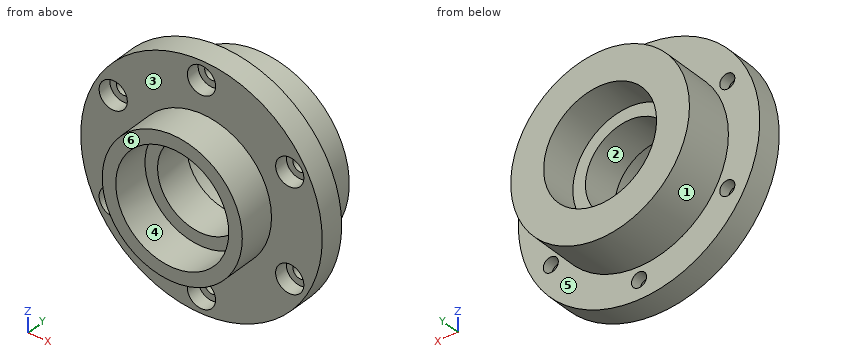
from build123d import *

# Parameters (mm, degrees)
F0_R            = 30.5435
F1_DEPTH        = 6.35
F2_R            = 17.7165
F2_R_2          = 14.2875
F3_DEPTH        = 9.525
F4_R            = 22.606
F5_DEPTH        = 12.7
F6_R            = 14.2875
F7_DEPTH        = 9.525
F8_R            = 11.1125
F9_DEPTH        = 19.05
F11_D           = 3.81
F11_CBORE_D     = 7.1374
F11_CBORE_DEPTH = 3.5052


with BuildPart() as f1:
    # F0 (on Front) → F1 (new body)
    with BuildSketch(Plane.XZ):
        Circle(F0_R)
    extrude(amount=F1_DEPTH)

    # F2 (on face) → F3 (join)
    with BuildSketch(Plane.XZ.offset(6.35)):
        Circle(F2_R)
        Circle(F2_R_2, mode=Mode.SUBTRACT)
    extrude(amount=F3_DEPTH)

    # F4 (on face) → F5 (join)
    with BuildSketch(Plane(origin=(0, 0, 0), x_dir=(-1, 0, 0), z_dir=(0, 1, 0))):
        Circle(F4_R)
    extrude(amount=F5_DEPTH)

    # F6 (on face) → F7 (cut)
    with BuildSketch(Plane(origin=(0, 12.7, 0), x_dir=(-1, 0, 0), z_dir=(0, 1, 0))):
        Circle(F6_R)
    extrude(amount=-F7_DEPTH, mode=Mode.SUBTRACT)

    # F8 (on face) → F9 (cut, symmetric)
    with BuildSketch(Plane(origin=(0, 3.175, 0), x_dir=(-1, 0, 0), z_dir=(0, 1, 0))):
        Circle(F8_R)
    extrude(amount=F9_DEPTH, both=True, mode=Mode.SUBTRACT)

    # F11 (through all)
    with Locations(Plane.XZ.offset(6.35)):
        with Locations((0, 25.781), (-22.327000935, 12.8905), (-22.327000935, -12.8905), (0, -25.781), (22.327000935, -12.8905), (22.327000935, 12.8905)):
            CounterBoreHole(F11_D / 2, F11_CBORE_D / 2, F11_CBORE_DEPTH)


solid = f1.part
Build history of the part. All positions in model axes, mm. Face numbers are marked on the shaded views. A direction names the side the tool comes from. Round coordinates to 2 decimals unless told otherwise and drop trailing zeros. Write each loop counter-clockwise with the first axis right and the second up, starting at its lowest first coordinate (ties: lowest second). Pieces come first, ordered by that corner, then holes. Notation, with made-up numbers: M 0,18.25 L 17,18.25 A20 ccw 17,46.25 Z; hole C 53,36 d1. An arc over 180 degrees is marked long. Use CSV: the item, a comma, the result in double quotes.
1. Saw through at C-C (y = 0.75). Give the cut face in (x, z) (1 decimal).
Reply:
outline,"C 0,0 d45.2; hole C 0,0 d22.2"
2. Saw through at B-B (x = -6). Give the cut face in (y, z) (3 decimals).
Reply:
outline,"M -15.875,-16.67 L -6.35,-16.67 L -6.35,-29.948 L 0,-29.948 L 0,-21.795 L 12.7,-21.795 L 12.7,-12.967 L 3.175,-12.967 L 3.175,-9.353 L -6.35,-9.353 L -6.35,-12.967 L -15.875,-12.967 Z; M -15.875,12.967 L -6.35,12.967 L -6.35,9.353 L 3.175,9.353 L 3.175,12.967 L 12.7,12.967 L 12.7,21.795 L 0,21.795 L 0,29.948 L -6.35,29.948 L -6.35,16.67 L -15.875,16.67 Z"
3. Flat gauge pins, fed straight in: pin 1 (8 mm diameter, centred on x = 21.5, z = 13, fed in from -Y); pin 2 (4.5 mm diameter, centred on x = 22.33, z = -12.89, fed in from -Y); pin 3 (12 mm diameter, centred on y = 9, z = 0, fed in from -X). Where does each tip first touch, or does it go through?
Reply:
pin 1,"stops at y = -6.35"
pin 2,"stops at y = -2.84"
pin 3,"stops at x = -22.61"
4. Tool access for the marked faces 4, 5 and 6: list every direction of +Z, -Z, +X, -X, +Y, -Y with a clear straight run to the whole face (end or side of a thin tool).
Reply:
face 4,"-Y"
face 5,"+Y"
face 6,"+Z, -Z, +X, -X, -Y"
5. Two-plate mould, pull along Z, no slides. Class the marked faces 1, 2 and 3: +Z half, -Z half, draft (parallel to the pull), parting line (faces both ways), or undercut.
Reply:
face 1,"parting line"
face 2,"undercut"
face 3,"draft"
6. Saw through at D-D (x = 12). Give the cut face in (y, z) (3 decimals).
Reply:
outline,"M -15.875,-13.034 L -6.35,-13.034 L -6.35,-28.087 L 0,-28.087 L 0,-19.158 L 12.7,-19.158 L 12.7,-7.755 L 3.175,-7.755 L 3.175,7.755 L 12.7,7.755 L 12.7,19.158 L 0,19.158 L 0,28.087 L -6.35,28.087 L -6.35,13.034 L -15.875,13.034 L -15.875,7.755 L -6.35,7.755 L -6.35,-7.755 L -15.875,-7.755 Z"
7. Wall check: probe 1 along Z at (x, y) = (0, -1.7); probe 2 along Z at (x, y) = (0, 10.5); probe 3 along Z at (x, y) = (0, -3). Give the ranges that are in metal, low to high. Write a range as from..to.
Reply:
probe 1,"z = -30.54..-27.69, -23.88..-11.11, 11.11..23.88, 27.69..30.54"
probe 2,"z = -22.61..-14.29, 14.29..22.61"
probe 3,"z = -30.54..-29.35, -22.21..-11.11, 11.11..22.21, 29.35..30.54"
